Read the model definition and answer for the solid it produces. Units are mm, in the model's axes. Face numbers are marked on the shaded views. A direction names the side the tool comes from. Coordinates: 2 decimals unless noted, no trailing zeros. Write each loop counter-clockwise with the first axis right and the second up, starting at its lowest first coordinate (ties: lowest second). Pieces come first, ordered by that corner, then holes. Notation, with made-up numbers: (42, 80) - (60, 80) arc R10 ccw to (60, 90) - close; hole circle Ø10 at (-16, -28.5). An arc over 180 degrees is marked (long way). Use a Markdown table: item, result.
from build123d import *

# Parameters (mm, degrees)
SKETCH_1_R          = 18.25
SKETCH_1_R_2        = 1.6
SKETCH_1_R_3        = 0.9
EXTRUDE_1_DEPTH     = 4
SKETCH_2_W          = 37
SKETCH_2_H          = 4
EXTRUDE_2_DEPTH     = 25
SKETCH_3_R          = 1.6
CUT_EXTRUDE_1_DEPTH = 72.716563183


with BuildPart() as part:
    # 草图1 → 凸台-拉伸1 (new body)
    with BuildSketch(Plane.XY):
        with BuildLine():
            Line((-18.5, -34), (18.5, -34))
            Line((18.5, -34), (18.5, -30))
            Line((18.5, -30), (27, -21.5))
            Line((27, -21.5), (29.5, -21.5))
            Line((29.5, -21.5), (29.5, 21.5))
            Line((29.5, 21.5), (27, 21.5))
            ThreePointArc((27, 21.5), (0, 28.583405797), (-27, 21.5))
            Line((-27, 21.5), (-29.5, 21.5))
            Line((-29.5, 21.5), (-29.5, -21.5))
            Line((-29.5, -21.5), (-27, -21.5))
            Line((-27, -21.5), (-18.5, -30))
            Line((-18.5, -30), (-18.5, -34))
        make_face()
        Circle(SKETCH_1_R, mode=Mode.SUBTRACT)
        with Locations((0, 25)):
            Circle(SKETCH_1_R_2, mode=Mode.SUBTRACT)
        with Locations((21.650635095, -12.5)):
            Circle(SKETCH_1_R_2, mode=Mode.SUBTRACT)
        with Locations((-21.650635095, -12.5)):
            Circle(SKETCH_1_R_2, mode=Mode.SUBTRACT)
        with Locations((-15, 17)):
            Circle(SKETCH_1_R_3, mode=Mode.SUBTRACT)
        with Locations(Location((15, 17, 0), (0, 0, 180))):
            Circle(SKETCH_1_R_3, mode=Mode.SUBTRACT)
        with Locations((15, -17)):
            Circle(SKETCH_1_R_3, mode=Mode.SUBTRACT)
        with Locations(Location((-15, -17, 0), (0, 0, 180))):
            Circle(SKETCH_1_R_3, mode=Mode.SUBTRACT)
    extrude(amount=EXTRUDE_1_DEPTH)

    # 草图2 → 凸台-拉伸2 (add)
    with BuildSketch(Plane.XY.offset(4)):
        with Locations((0, -32)):
            Rectangle(SKETCH_2_W, SKETCH_2_H)
    extrude(amount=EXTRUDE_2_DEPTH)

    # 草图3 → 切除-拉伸1 (cut, through all)
    with BuildSketch(Plane(origin=(0, -30, 0), x_dir=(1, 0, 0), z_dir=(0, 1, 0))):
        with Locations(Location((-6, -16.5, 0), (0, 0, 180))):
            Circle(SKETCH_3_R)
        with Locations((6, -16.5)):
            Circle(SKETCH_3_R)
    extrude(amount=-CUT_EXTRUDE_1_DEPTH, mode=Mode.SUBTRACT)


solid = part.part
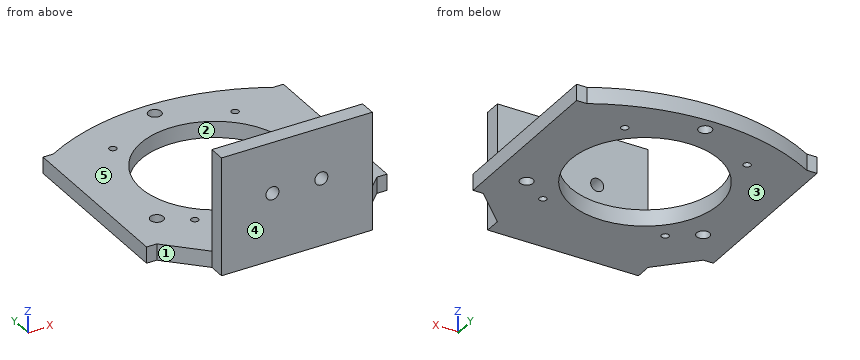
(1) Each of these flat-tipped pins is pushed along its axis until it touches: P1, Ø3, axis at x = 22.5, z = 3, coming from the -Y side; P2, Ø1.2, axis at x = -28.5, z = 2.5, coming from the -Y side; P3, Ø4, axis at x = 0, y = 25, coming from the +Z side. Where does it stop, or does it pass through?
Report:
| item | result |
|---|---|
| P1 | stops at y = -27.5 |
| P2 | stops at y = -21.5 |
| P3 | stops at z = 4 |
(2) A cutting plane is placed at B-B, the plane x = 0. Write down the section's boundary in (y, z), and give its area (3 significant figures).
Report:
| item | result |
|---|---|
| outline | (-34, 0) - (-18.25, 0) - (-18.25, 4) - (-30, 4) - (-30, 29) - (-34, 29) - close; (18.25, 0) - (23.4, 0) - (23.4, 4) - (18.25, 4) - close; (26.6, 0) - (28.58, 0) - (28.58, 4) - (26.6, 4) - close |
| area | 192 mm² |
(3) Straight lines are drawn through the part: L1, parallel to Z at x = 6, y = -30.8; L2, parallel to Y at x = 0, z = 1.25; L3, parallel to Y at x = 5.5, z = 6.5. For each, find the intervals that lie inside material, in ascending order.
Report:
| item | result |
|---|---|
| L1 | z = 0 to 14.9, 18.1 to 29 |
| L2 | y = -34 to -18.25, 18.25 to 23.4, 26.6 to 28.58 |
| L3 | y = -34 to -30 |
(4) A cutting plane is placed at D-D, the plane x = 12.5. Write down the section's boundary in (y, z).
Report:
| item | result |
|---|---|
| outline | (-34, 0) - (-13.3, 0) - (-13.3, 4) - (-30, 4) - (-30, 29) - (-34, 29) - close; (13.3, 0) - (27.14, 0) - (27.14, 4) - (13.3, 4) - close |
(5) For the marked faces 4 and 5, determine the directions among +Z, -Z, +X, -X, +Y, -Y from which every point of the face is accessible in a straight line to the end or side of a thin tool.
Report:
| item | result |
|---|---|
| face 4 | +Z, -Z, +X, -X, -Y |
| face 5 | +Z, +X, -X, +Y |
(6) A cutting plane is placed at A-A, the plane z = 16.5. Write down the section's boundary in (x, y), and give its area (3 significant figures).
Report:
| item | result |
|---|---|
| outline | (-18.5, -34) - (-7.6, -34) - (-7.6, -30) - (-18.5, -30) - close; (-4.4, -34) - (4.4, -34) - (4.4, -30) - (-4.4, -30) - close; (7.6, -34) - (18.5, -34) - (18.5, -30) - (7.6, -30) - close |
| area | 122 mm² |
(7) A cutting plane is placed at C-C, the plane y = 25. Write down the section's boundary in (x, z).
Report:
| item | result |
|---|---|
| outline | (-19.53, 0) - (-1.6, 0) - (-1.6, 4) - (-19.53, 4) - close; (1.6, 0) - (19.53, 0) - (19.53, 4) - (1.6, 4) - close |
(8) The mould has two halves that part along X. Classify the marked faces 1, 2 and 3: pulls with the +X half, pulls with the -X half, needs draft (parallel to the pull), parting line crosses it, or undercut.
Report:
| item | result |
|---|---|
| face 1 | pulls with the -X half |
| face 2 | undercut |
| face 3 | needs draft |
